CAD build for the part. Positions are in the model's coordinates, mm. A direction names the side the tool comes from. Give positions to 0.01 mm unless a question says otherwise; leave off trailing zeros. Loops run counter-clockwise (first coordinate to the right, second up) from the corner with the lowest first, then second, coordinate; pieces in that order, holes last.
```python
from build123d import *

# Parameters (mm, degrees)
SKETCH1_R           = 20
BOSS_EXTRUDE1_DEPTH = 20
SKETCH2_R           = 17.5
SKETCH2_R_2         = 15
CUT_EXTRUDE1_DEPTH  = 10
CUT_EXTRUDE1_TAPER  = 20
SKETCH3_R           = 2
CUT_EXTRUDE2_DEPTH  = 5


with BuildPart() as part:
    # Sketch1 → Boss-Extrude1 (new body)
    with BuildSketch(Plane(origin=(0, 0, 0), x_dir=(1, 0, 0), z_dir=(0, 1, 0))):
        with Locations(Location((0, 0, 0), (0, 0, 270))):
            Circle(SKETCH1_R)
    extrude(amount=BOSS_EXTRUDE1_DEPTH)

    # Sketch2 → Cut-Extrude1 (cut)
    with BuildSketch(Plane(origin=(0, 20, 0), x_dir=(1, 0, 0), z_dir=(0, 1, 0))):
        Circle(SKETCH2_R)
        Circle(SKETCH2_R_2, mode=Mode.SUBTRACT)
    extrude(amount=-CUT_EXTRUDE1_DEPTH, taper=CUT_EXTRUDE1_TAPER, mode=Mode.SUBTRACT)

    # Sketch3 → Cut-Extrude2 (cut)
    with BuildSketch(Plane.XZ):
        with Locations(Location((0, 0, 0), (0, 0, 270))):
            Circle(SKETCH3_R)
    extrude(amount=-CUT_EXTRUDE2_DEPTH, mode=Mode.SUBTRACT)


solid = part.part
```
1. Probe line 1 along X through (y, z) = (2.7, 0); line 2 along Z through (x, y) = (-2, 17.25); line 3 along Z through (x, y) = (1, 3). List the from-to ranges inside material, lowest first.
Responses:
line 1: x = -20 to -2, 2 to 20
line 2: z = -19.9 to -16.38, -15.88 to 15.88, 16.38 to 19.9
line 3: z = -19.97 to -1.73, 1.73 to 19.97
2. Saw through at B-B, the plane y = 8. List the corners of the cut face in (x, z).
Responses:
outline: circle Ø40 at (0, 0)
3. Saw through at A-A, the plane x = 0. List the corners of the cut face in (y, z).
Responses:
outline: (0, -20) - (20, -20) - (20, -17.5) - (16.57, -16.25) - (20, -15) - (20, 15) - (16.57, 16.25) - (20, 17.5) - (20, 20) - (0, 20) - (0, 2) - (5, 2) - (5, -2) - (0, -2) - close
4. Tool access for faces 1 (the face through (-18, 20, 0)), 2 (the face through (0, 5, 0)): list every direction of +Z, -Z, +X, -X, +Y, -Y with a clear straight run to the whole face (end or side of a thin tool).
Responses:
face 1: +Z, -Z, +X, -X, +Y
face 2: -Y
5. Drop flat-ended pins along their axis: pin 1 (6 mm diameter, centred on x = -13, z = 11, fed in from +Y); pin 2 (2 mm diameter, centred on y = 16.5, z = -10.5, fed in from +X); pin 3 (8 mm diameter, centred on y = 17.5, z = 5, fed in from -X) (3 decimals); pin 4 (1 mm diameter, centred on y = 13, z = -15, fed in from +X) (3 decimals). Give the stop position or say it passes through.
Responses:
pin 1: stops at y = 20
pin 2: stops at x = 17.6
pin 3: stops at x = -19.975
pin 4: stops at x = 13.775
6. Pull direction Z, two halves, no side cores. Call faces 3 (the face through (-19.524, 9.86, -4.336)), 4 (the face through (0, 0, 4)), 5 (the face through (-2, 2, 0)): released by +Z, released by -Z, zero draft, split by the parting line, or undercut.
Responses:
face 3: split by the parting line
face 4: zero draft
face 5: undercut
7. Saw through at D-D, the plane y = 4.25. List the corners of the cut face in (x, z), and give its area (3 significant figures).
Responses:
outline: circle Ø40 at (0, 0); hole circle Ø4 at (0, 0)
area: 1,240 mm2
8. Saw through at C-C, the plane y = 17.5. List the corners of the cut face in (x, z), and give its area (3 significant figures).
Responses:
outline: circle Ø40 at (0, 0); circle Ø31.82 at (0, 0); hole circle Ø33.18 at (0, 0)
area: 1,190 mm2
